Part model, mm, in its own coordinate system. Round coordinates to 2 decimals unless told otherwise and drop trailing zeros. Order: outer loops, then holes, each group sorted by start corner. A loop starts at its lowest first (then second) coordinate and runs counter-clockwise, first axis right, second up. Notation, with made-up numbers: (-30.75, 34.5) - (-1.75, 34.5) arc R14 cw to (-1.75, 44.5) - close; hole circle Ø4 at (-25.75, -34). An arc over 180 degrees is marked (long way). Return JSON: item names as keys, results as strings. Group by question number.
Item 1: Saw through at B-B on z = 0.55. State how many separate pieces and enclosed holes the cut face has, and give its area (3 significant figures).
Item 2: Probe probe 1 along X at (y, z) = (-3, 0.85); probe 2 along X at (y, z) = (2.5, 0.9); probe 3 along X at (y, z) = (-11, 0.45). List the from-to ranges inside material, lowest first.
Item 3: Saw through at A-A on x = 0. List the corners of the cut face in (y, z) (1 decimal), and give its area (3 significant figures).
Item 4: Saw through at C-C on x = -93.5. List the corners of the cut face in (y, z) (3 decimals), and give its area (3 significant figures).
Item 5: Saw through at D-D on x = -522. List the corners of the cut face in (y, z) (3 decimals).
Item 6: Drop flat-ended pins along their axis: pin 1 (3 mm diameter, centred on x = -514.47, y = -32.91, fed in from +Z); pin 2 (1 mm diameter, centred on y = -17.5, z = 2, fed in from +X). Give the stop position or say it passes through.
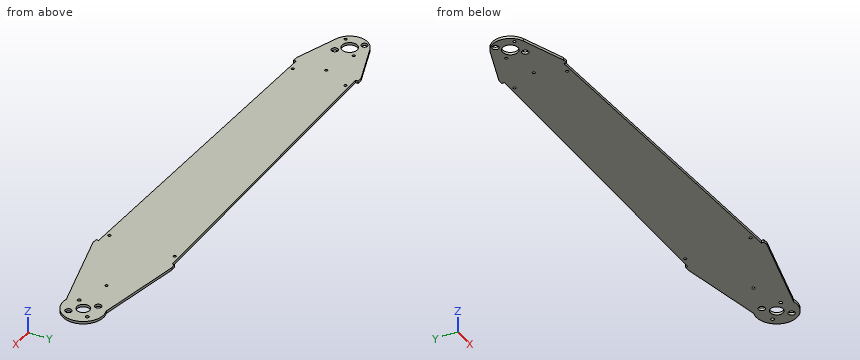
```python
from build123d import *

# Parameters (mm, degrees)
F0_R     = 1.7272
F0_R_2   = 3.96875
F0_R_3   = 2.15265
F0_R_4   = 9.525
F0_R_5   = 7.9375
F1_DEPTH = 3.175


with BuildPart() as f1:
    # F0 (on Top) → F1 (new body)
    with BuildSketch(Plane.XY):
        with BuildLine():
            Line((-535.358043, 40.160772), (-588.318702, 20.884668))
            ThreePointArc((-588.318702, 20.884668), (-602.942304, 0), (-588.318702, -20.884668))
            Line((-588.318702, -20.884668), (-535.358043, -40.160772))
            Line((-535.358043, -40.160772), (-529.011557, -40.371983))
            Line((-529.011557, -40.371983), (-528.905951, -37.19874))
            Line((-528.905951, -37.19874), (-122.326798, -50.729687))
            Line((-122.326798, -50.729687), (-122.432403, -53.90293))
            Line((-122.432403, -53.90293), (-116.085917, -54.114141))
            Line((-116.085917, -54.114141), (-6.125468, -24.650327))
            ThreePointArc((-6.125468, -24.650327), (25.380331, 0.99941), (-8.044825, 24.092339))
            Line((-8.044825, 24.092339), (-115.871895, 44.057476))
            Line((-115.871895, 44.057476), (-122.221621, 43.998492))
            Line((-122.221621, 43.998492), (-122.192129, 40.823629))
            Line((-122.192129, 40.823629), (-528.978825, 37.044893))
            Line((-528.978825, 37.044893), (-529.008317, 40.219756))
            Line((-529.008317, 40.219756), (-535.358043, 40.160772))
        make_face()
        with Locations((-514.467949, -32.914099)):
            Circle(F0_R, mode=Mode.SUBTRACT)
        with Locations((-592.503891, -11.786586)):
            Circle(F0_R, mode=Mode.SUBTRACT)
        with Locations((-568.930718, -11.786586)):
            Circle(F0_R_2, mode=Mode.SUBTRACT)
        with Locations((-136.447984, -45.494597)):
            Circle(F0_R, mode=Mode.SUBTRACT)
        with Locations((-11.786586, -11.786586)):
            Circle(F0_R_3, mode=Mode.SUBTRACT)
        with Locations((11.786586, -11.786586)):
            Circle(F0_R_2, mode=Mode.SUBTRACT)
        with Locations((-580.717304, 0)):
            Circle(F0_R_4, mode=Mode.SUBTRACT)
        with Locations((-529.917304, 0)):
            Circle(F0_R, mode=Mode.SUBTRACT)
        with Locations((-592.503891, 11.786586)):
            Circle(F0_R_2, mode=Mode.SUBTRACT)
        with Locations((-568.930718, 11.786586)):
            Circle(F0_R, mode=Mode.SUBTRACT)
        with Locations((-514.647704, 32.415313)):
            Circle(F0_R, mode=Mode.SUBTRACT)
        with Locations((-50.8, 0)):
            Circle(F0_R, mode=Mode.SUBTRACT)
        Circle(F0_R_5, mode=Mode.SUBTRACT)
        with Locations((-11.786586, 11.786586)):
            Circle(F0_R_2, mode=Mode.SUBTRACT)
        with Locations((11.786586, 11.786586)):
            Circle(F0_R_3, mode=Mode.SUBTRACT)
        with Locations((-136.434775, 35.92862)):
            Circle(F0_R, mode=Mode.SUBTRACT)
    extrude(amount=F1_DEPTH)


solid = f1.part
```
Filled in:
{
 "1": {"separate pieces": "1", "enclosed holes": "16", "area": "47,100 mm^2"},
 "2": {"probe 1": "x = -602.74 to -589.76, -571.68 to -7.35, 7.35 to 25.22", "probe 2": "x = -602.8 to -589.91, -571.53 to -7.53, 7.53 to 25.28", "probe 3": "x = -600.03 to -594.04, -590.97 to -572.82, -565.04 to -13.79, -9.78 to 7.9, 15.68 to 22.89"},
 "3": {"outline": "(-25.4, 0) - (-7.9, 0) - (-7.9, 3.2) - (-25.4, 3.2) - close; (7.9, 0) - (25.4, 0) - (25.4, 3.2) - (7.9, 3.2) - close", "area": "111 mm^2"},
 "4": {"outline": "(-48.062, 0) - (39.915, 0) - (39.915, 3.175) - (-48.062, 3.175) - close", "area": "279 mm^2"},
 "5": {"outline": "(-37.429, 0) - (37.11, 0) - (37.11, 3.175) - (-37.429, 3.175) - close"},
 "6": {"pin 1": "passes through", "pin 2": "stops at x = 18.87"}
}
